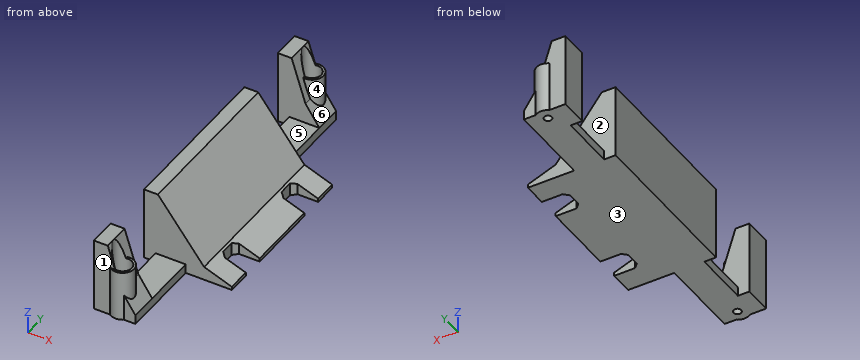
from build123d import *

# Parameters (mm, degrees)
F_4MM_DEPTH             = 4
F_6MM_0_START           = -36
F_6MM_0_DEPTH           = 72
F_6MM_66_START          = 60
F_6MM_66_DEPTH          = 12
F_6MM_66_START_2        = -72
F_6MM_66_2_DEPTH        = 12
SKETCH_5_R              = 1.65
CUT_EXTRUDE_M3_DEPTH    = 4
SKETCH_7_R              = 5
SKETCH_7_R_2            = 1.65
EXTRUDE_D10_DEPTH       = 22
D8_4MM_START            = 4
SKETCH_8_R              = 4
D8_4MM_DEPTH            = 32
CUT_EXTRUDE_14X10_DEPTH = 40


with BuildPart() as part:
    # 草图1 → 加厚侧鞍底梁_4mm (new body)
    with BuildSketch(Plane.XY):
        Polygon((37, -72), (46, -72), (48, -70), (48, 70), (46, 72), (37, 72), (35, 70), (35, -70), align=None)
    extrude(amount=F_4MM_DEPTH)

    # 草图2 → 高侧壁6mm_分段缓降斜面_0 (add)
    with BuildSketch(Plane(origin=(0, 0, 0), x_dir=(1, 0, 0), z_dir=(0, 1, 0)).offset(F_6MM_0_START)):
        Polygon((30, 0), (68, 0), (68, -1.5), (56, -6), (36, -32), (30, -32), align=None)
    extrude(amount=F_6MM_0_DEPTH)

    # 草图3 → 6mm___66 (add)
    with BuildSketch(Plane(origin=(0, 0, 0), x_dir=(1, 0, 0), z_dir=(0, 1, 0)).offset(F_6MM_66_START)):
        Polygon((30, 0), (48, 0), (48, -4), (42, -13), (36, -32), (30, -32), align=None)
    extrude(amount=F_6MM_66_DEPTH)

    # 草图4 → 6mm___-66 2 (add)
    with BuildSketch(Plane(origin=(0, 0, 0), x_dir=(1, 0, 0), z_dir=(0, 1, 0)).offset(F_6MM_66_START_2)):
        Polygon((30, 0), (48, 0), (48, -4), (42, -13), (36, -32), (30, -32), align=None)
    extrude(amount=F_6MM_66_2_DEPTH)

    # 草图5 → 侧鞍M3贯穿固定孔 (cut)
    with BuildSketch(Plane.XY):
        with Locations((40, -68)):
            Circle(SKETCH_5_R)
        with Locations((40, 68)):
            Circle(SKETCH_5_R)
    extrude(amount=CUT_EXTRUDE_M3_DEPTH, mode=Mode.SUBTRACT)

    # 草图7 → 螺丝沉台局部加强圈_D10 (add)
    # profile 1 of 2: a face of its own
    with BuildSketch(Plane.XY):
        with Locations((40, -68)):
            Circle(SKETCH_7_R)
        with Locations((40, -68)):
            Circle(SKETCH_7_R_2, mode=Mode.SUBTRACT)
    # profile 2 of 2: a face of its own
    with BuildSketch(Plane.XY):
        with Locations((40, 68)):
            Circle(SKETCH_7_R)
        with Locations((40, 68)):
            Circle(SKETCH_7_R_2, mode=Mode.SUBTRACT)
    extrude(amount=EXTRUDE_D10_DEPTH)

    # 草图8 → 螺丝头及工具沉台_D8_保留4mm底 (cut)
    with BuildSketch(Plane.XY.offset(D8_4MM_START)):
        with Locations(Location((40, -68, 0), (0, 0, 180))):
            Circle(SKETCH_8_R)
        with Locations(Location((40, 68, 0), (0, 0, 180))):
            Circle(SKETCH_8_R)
    extrude(amount=D8_4MM_DEPTH, mode=Mode.SUBTRACT)

    # 草图9 → 板内钢索孔侧向敞口避让_14x10 (cut)
    with BuildSketch(Plane.XY):
        Polygon((59, 16), (69, 16), (71, 18), (71, 24), (69, 26), (59, 26), (57, 24), (57, 18), align=None)
        Polygon((59, -26), (69, -26), (71, -24), (71, -18), (69, -16), (59, -16), (57, -18), (57, -24), align=None)
    extrude(amount=CUT_EXTRUDE_14X10_DEPTH, mode=Mode.SUBTRACT)


solid = part.part
Can you work these out from the model? Positions are in its coordinate system, mm. Face numbers are marked on the shaded views. A direction names the side the tool comes from. Coordinates: 2 decimals unless noted, no trailing zeros. Write each loop counter-clockwise with the first axis right and the second up, starting at its lowest first coordinate (ties: lowest second). Pieces come first, ordered by that corner, then holes. Notation, with made-up numbers: (-34, 84.25) -> (15, 84.25) arc R22 ccw to (15, 119.25) -> close; hole circle Ø8 at (8.25, 21). An arc over 180 degrees is marked (long way). Answer as CSV lines item,"result".
1) On a 3-axis mill with a long thin cutter (end or side, diameter ignored), from which of +Z, -Z, +X, -X, +Y, -Y can I reach the whole of each face in a straight line? I mean the marked faces 4, 5 and 6. Say none if no direction works.
Check result:
face 4,"+Z"
face 5,"+Z, +X, -X"
face 6,"+Z, +X"
2) Will these pins go through, and if not, where does the flat tip stop? P1, Ø2.5, axis at x = 39, y = -67, coming from the +Z side; P2, Ø4, axis at x = 46.5, z = 3.5, coming from the -Y side; P3, Ø4, axis at y = 17, z = 16.5, coming from the +X side.
Check result:
P1,"z = 4"
P2,"y = -72"
P3,"x = 49.46"
3) If we section it at A-A on z = 16.5: Please give me the cut outline in (x, y).
Check result:
outline,"(30, -72) -> (37, -72) arc R5 ccw (long way) to (40.89, -63.08) -> (40.89, -60) -> (30, -60) -> close; (30, -36) -> (47.92, -36) -> (47.92, 36) -> (30, 36) -> close; (30, 60) -> (40.89, 60) -> (40.89, 63.08) arc R5 ccw (long way) to (37, 72) -> (30, 72) -> close; hole circle Ø8 at (40, -68); hole circle Ø8 at (40, 68)"
4) If we section it at C-C on y = 12.5: Please give me the cut outline in (x, z), then the cut area to 3 significant figures.
Check result:
outline,"(30, 0) -> (68, 0) -> (68, 1.5) -> (56, 6) -> (36, 32) -> (30, 32) -> close"
area,"617 mm²"
5) If I drill on line 1 (Y direction, x = 40, z = 20); line 2 (Y direction, x = 40, z = 1); line 3 (Y direction, x = 32.5, z = 4), over which ranges is the centre line in solid material (lowest first)? Write a range as from..to.
Check result:
line 1,"-73..-72, -64..-63, -36..36, 63..64, 72..73"
line 2,"-73..-69.65, -66.35..66.35, 69.65..73"
line 3,"-72..-60, -36..36, 60..72"
6) If we section it at B-B on z = 24: Please give me the cut outline in (x, y).
Check result:
outline,"(30, -72) -> (38.53, -72) -> (38.53, -71.72) arc R4 cw to (38.53, -64.28) -> (38.53, -60) -> (30, -60) -> close; (30, -36) -> (42.15, -36) -> (42.15, 36) -> (30, 36) -> close; (30, 60) -> (38.53, 60) -> (38.53, 64.28) arc R4 cw to (38.53, 71.72) -> (38.53, 72) -> (30, 72) -> close"
7) If we mould it in two halves opening along Y, with no side actions, what happens to the marked faces 1, 2 and 3? For each: +Y half, -Y half, draft (parallel to the pull), parting line (faces both ways), or undercut.
Check result:
face 1,"-Y half"
face 2,"undercut"
face 3,"draft"
